Build history of the part. All positions in model axes, mm. Face numbers are marked on the shaded views. A direction names the side the tool comes from. Round coordinates to 2 decimals unless told otherwise and drop trailing zeros. Write each loop counter-clockwise with the first axis right and the second up, starting at its lowest first coordinate (ties: lowest second). Pieces come first, ordered by that corner, then holes.
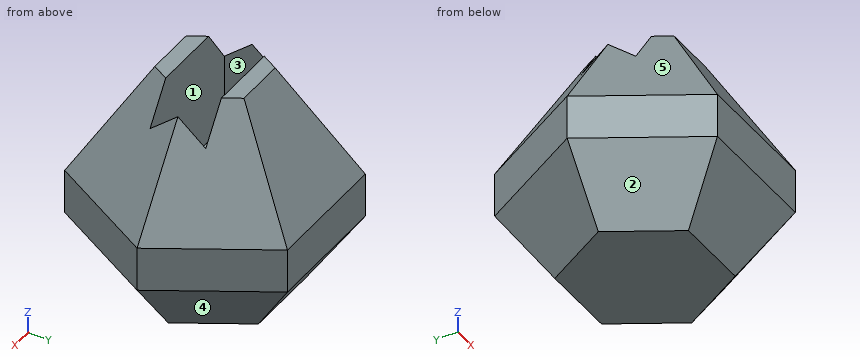
from build123d import *

# Parameters (mm, degrees)
F0_W        = 5.5
F0_H        = 2.5
F1_DEPTH    = 10
F2_T1_DEPTH = 21.2763058351
F2_T3_DEPTH = 21.2763058351
F2_T5_DEPTH = 21.2763058351
F2_T7_DEPTH = 21.2763058351
F2_T9_DEPTH = 21.2763058351
F3_T1_DEPTH = 31.6361136638
F3_T3_DEPTH = 31.6361136638
F3_T5_DEPTH = 31.6361136638
F3_T7_DEPTH = 31.6361136638
F3_T9_DEPTH = 31.6361136638
F4_DEPTH    = 5


# Not quite as in the source:
# - a fillet or chamfer that OpenCascade refuses, or shapes differently, is made with other operations: its cross-section is extruded or revolved along the edge and cut away or added


with BuildPart() as f1:
    # F0 (on Top) → F1 (new body)
    with BuildSketch(Plane.XY):
        Polygon((2.8867513459, 5), (-2.8867513459, 5), (-5.7735026919, 0), (-2.8867513459, -5), (2.8867513459, -5), (5.7735026919, 0), align=None)
        Rectangle(F0_W, F0_H, mode=Mode.SUBTRACT)
    extrude(amount=F1_DEPTH)

    # F2: chamfer of 2 x 3 on 6 edges, made by hand

    # F2_s2 → F2_t1 (cut)
    with BuildSketch(Plane.YZ.offset(-10.6381529176)):
        Polygon((5, 3), (3, 0), (5, 0), align=None)
        Polygon((-5, 3), (-3, 0), (-5, 0), align=None)
    extrude(amount=F2_T1_DEPTH, mode=Mode.SUBTRACT)

    # F2_s4 → F2_t3 (cut)
    with BuildSketch(Plane(origin=(5.3190764588, -9.212910676, 0), x_dir=(0, 0, 1), z_dir=(-0.5, 0.8660254038, 0))):
        Polygon((3, 5), (0, 3), (0, 5), align=None)
    extrude(amount=F2_T3_DEPTH, mode=Mode.SUBTRACT)

    # F2_s6 → F2_t5 (cut)
    with BuildSketch(Plane(origin=(5.3190764588, 9.212910676, 0), x_dir=(0, 0, 1), z_dir=(-0.5, -0.8660254038, 0))):
        Polygon((3, 5), (0, 3), (0, 5), align=None)
    extrude(amount=F2_T5_DEPTH, mode=Mode.SUBTRACT)

    # F2_s8 → F2_t7 (cut)
    with BuildSketch(Plane(origin=(-5.3190764588, 9.212910676, 0), x_dir=(0, 0, 1), z_dir=(0.5, -0.8660254038, 0))):
        Polygon((3, 5), (0, 3), (0, 5), align=None)
    extrude(amount=F2_T7_DEPTH, mode=Mode.SUBTRACT)

    # F2_s10 → F2_t9 (cut)
    with BuildSketch(Plane(origin=(-5.3190764588, -9.212910676, 0), x_dir=(0, 0, 1), z_dir=(0.5, 0.8660254038, 0))):
        Polygon((3, 5), (0, 3), (0, 5), align=None)
    extrude(amount=F2_T9_DEPTH, mode=Mode.SUBTRACT)

    # F3: chamfer of 5 x 3 on 6 edges, made by hand

    # F3_s2 → F3_t1 (cut)
    with BuildSketch(Plane(origin=(7.909028416, -13.6988390549, 0), x_dir=(0, 0, 1), z_dir=(-0.5, 0.8660254038, 0))):
        Polygon((5, 5), (10, 2), (10, 5), align=None)
    extrude(amount=F3_T1_DEPTH, mode=Mode.SUBTRACT)

    # F3_s4 → F3_t3 (cut)
    with BuildSketch(Plane.YZ.offset(-15.8180568319)):
        Polygon((5, 5), (2, 10), (5, 10), align=None)
        Polygon((-2, 10), (-5, 5), (-5, 10), align=None)
    extrude(amount=F3_T3_DEPTH, mode=Mode.SUBTRACT)

    # F3_s6 → F3_t5 (cut)
    with BuildSketch(Plane(origin=(7.909028416, 13.6988390549, 0), x_dir=(0, 0, 1), z_dir=(-0.5, -0.8660254038, 0))):
        Polygon((10, 2), (5, 5), (10, 5), align=None)
    extrude(amount=F3_T5_DEPTH, mode=Mode.SUBTRACT)

    # F3_s8 → F3_t7 (cut)
    with BuildSketch(Plane(origin=(-7.909028416, 13.6988390549, 0), x_dir=(0, 0, 1), z_dir=(0.5, -0.8660254038, 0))):
        Polygon((10, 2), (5, 5), (10, 5), align=None)
    extrude(amount=F3_T7_DEPTH, mode=Mode.SUBTRACT)

    # F3_s10 → F3_t9 (cut)
    with BuildSketch(Plane(origin=(-7.909028416, -13.6988390549, 0), x_dir=(0, 0, 1), z_dir=(0.5, 0.8660254038, 0))):
        Polygon((10, 2), (5, 5), (10, 5), align=None)
    extrude(amount=F3_T9_DEPTH, mode=Mode.SUBTRACT)

    # F0 (on Top) → F4 (join)
    with BuildSketch(Plane.XY):
        Rectangle(F0_W, F0_H)
    extrude(amount=F4_DEPTH)


solid = f1.part
1) Wall check: L1, parallel to Y at x = 2.25, z = 8.75; L2, parallel to X at y = 0.25, z = 8.5; L3, parallel to Y at x = -1, z = 7.5. Give the ranges that are in metal, low to high.
Results:
L1: y = -1.6 to -1.25, 1.25 to 1.6
L2: x = -3.2 to -2.75, 2.75 to 3.2
L3: y = -3.5 to -1.25, 1.25 to 3.5
2) Pin check, flat tips, straight feed: pin 1 Ø1 at (x, y) = (3, -3) entering from +Z; pin 2 Ø2.5 at (x, z) = (1, 7) entering from +Y; pin 3 Ø1.2 at (y, z) = (0, 7) entering from -X; pin 4 Ø4 at (x, y) = (-3, -2.5) entering from +Z. Stop position of each tip, or through.
Results:
pin 1: stops at z = 7.34
pin 2: stops at y = 4.55
pin 3: stops at x = -4.8
pin 4: stops at z = 10
3) Slice it at D-D (z = 7.5). Write the cut outline in (x, y).
Results:
outline: (-4.04, 0) - (-2.02, -3.5) - (2.02, -3.5) - (4.04, 0) - (2.02, 3.5) - (-2.02, 3.5) - close; hole (-2.75, -1.25) - (2.75, -1.25) - (2.75, 1.25) - (-2.75, 1.25) - close
4) Slice it at C-C (y = -1.75). Write the cut outline in (x, z), plus the area to 3 significant figures.
Results:
outline: (-4.76, 3) - (-2.45, 0) - (2.45, 0) - (4.76, 3) - (4.76, 5) - (1.3, 10) - (-1.3, 10) - (-4.76, 5) - close
area: 71.0 mm2
5) Mould opens along X. For the marked faces 3, 4 and 5 say: released by +X, released by -X, zero draft, split by the parting line, or undercut.
Results:
face 3: undercut
face 4: released by +X
face 5: released by -X
6) Slice it at A-A (x = -0.75). Write the cut outline in (y, z).
Results:
outline: (-5, 3) - (-3, 0) - (3, 0) - (5, 3) - (5, 5) - (2, 10) - (1.25, 10) - (1.25, 5) - (-1.25, 5) - (-1.25, 10) - (-2, 10) - (-5, 5) - close
7) Which spindle directions (+Z, -Z, +X, -X, +Y, -Y) get a long thin tool onto all of the face, cutting with end or side? Do the marked faces 1 and 2. Say none if no direction does.
Results:
face 1: +Z
face 2: -Z, -X, -Y
8) Slice it at B-B (z = 4.25). Write the cut outline in (x, y).
Results:
outline: (-5.77, 0) - (-2.89, -5) - (2.89, -5) - (5.77, 0) - (2.89, 5) - (-2.89, 5) - close
